from build123d import *

# Parameters (mm, degrees)
SKETCH1_W           = 38.1
SKETCH1_H           = 38.1
BOSS_EXTRUDE1_DEPTH = 7.62
SKETCH2_R           = 19.05
BOSS_EXTRUDE2_DEPTH = 25.4
SKETCH3_W           = 38.1
SKETCH3_H           = 38.1
BOSS_EXTRUDE3_DEPTH = 15.24
SKETCH4_R           = 6.296459426
BOSS_EXTRUDE4_DEPTH = 76.2
SKETCH5_W           = 3.175
SKETCH5_H           = 1.58699954
CUT_EXTRUDE1_DEPTH  = 73.66
SKETCH6_R           = 2.54
SKETCH6_R_2         = 2.5
CUT_EXTRUDE2_DEPTH  = 7.62
BOSS_EXTRUDE5_START = 71.374
SKETCH7_R           = 19.05
BOSS_EXTRUDE5_DEPTH = 71.374


with BuildPart() as part:
    # Sketch1 → Boss-Extrude1 (new body)
    with BuildSketch(Plane(origin=(0, 0, 0), x_dir=(1, 0, 0), z_dir=(0, 1, 0))):
        Rectangle(SKETCH1_W, SKETCH1_H)
    extrude(amount=BOSS_EXTRUDE1_DEPTH)

    # Sketch2 → Boss-Extrude2 (add)
    with BuildSketch(Plane(origin=(0, 7.62, 0), x_dir=(1, 0, 0), z_dir=(0, 1, 0))):
        with Locations(Location((0, 0, 0), (0, 0, 270))):
            Circle(SKETCH2_R)
    extrude(amount=BOSS_EXTRUDE2_DEPTH)

    # Sketch3 → Boss-Extrude3 (add)
    with BuildSketch(Plane(origin=(0, 33.02, 0), x_dir=(1, 0, 0), z_dir=(0, 1, 0))):
        Rectangle(SKETCH3_W, SKETCH3_H)
    extrude(amount=BOSS_EXTRUDE3_DEPTH)

    # Sketch4 → Boss-Extrude4 (add)
    with BuildSketch(Plane(origin=(0, 48.26, 0), x_dir=(1, 0, 0), z_dir=(0, 1, 0))):
        with Locations(Location((0, 0, 0), (0, 0, 90))):
            Circle(SKETCH4_R)
    extrude(amount=BOSS_EXTRUDE4_DEPTH)

    # Sketch5 → Cut-Extrude1 (cut)
    with BuildSketch(Plane(origin=(0, 124.46, 0), x_dir=(1, 0, 0), z_dir=(0, 1, 0))):
        with Locations((0, 6.38149977)):
            Rectangle(SKETCH5_W, SKETCH5_H)
    extrude(amount=-CUT_EXTRUDE1_DEPTH, mode=Mode.SUBTRACT)

    # Fillet1: read off the stored shape, not the designer's step
    # Fillet1 outline → Fillet1 (revolve, cut)
    with BuildSketch(Plane.XY):
        with BuildLine():
            ThreePointArc((5.026459426, 124.46), (5.924485038, 124.088025612), (6.296459426, 123.19))
            Line((6.296459426, 123.19), (6.296459426, 124.46))
            Line((6.296459426, 124.46), (5.026459426, 124.46))
        make_face()
    revolve(axis=Axis((0, 0, 0), (0, 1, 0)), mode=Mode.SUBTRACT)

    # Sketch6 → Cut-Extrude2 (cut)
    with BuildSketch(Plane(origin=(0, 0, -19.05), x_dir=(-1, 0, 0), z_dir=(0, 0, -1))):
        with Locations((-9.525, 3.81)):
            Circle(SKETCH6_R)
        with Locations((-9.525, 40.64)):
            Circle(SKETCH6_R)
        with Locations((9.525, 40.64)):
            Circle(SKETCH6_R)
        with Locations((9.525, 3.81)):
            Circle(SKETCH6_R_2)
    cut_extrude2 = extrude(amount=-CUT_EXTRUDE2_DEPTH, mode=Mode.SUBTRACT)

    # Mirror1: Cut-Extrude2 across plane
    add(cut_extrude2.mirror(Plane.XY), mode=Mode.SUBTRACT)

    # Sketch7 → Boss-Extrude5 (add)
    with BuildSketch(Plane.XZ.offset(BOSS_EXTRUDE5_START)):
        with Locations(Location((0, 0, 0), (0, 0, 270))):
            Circle(SKETCH7_R)
    extrude(amount=-BOSS_EXTRUDE5_DEPTH)


solid = part.part
The listing builds one solid part. Answer for the finished solid, in the listing's coordinates (mm). A direction names the side the tool comes from. Coordinates: 2 decimals unless noted, no trailing zeros. Write each loop counter-clockwise with the first axis right and the second up, starting at its lowest first coordinate (ties: lowest second). Pieces come first, ordered by that corner, then holes. Notation, with made-up numbers: M 81.5,28 L 99.5,28 A24 ccw 99.5,51 Z; hole C 48,83 d6. An arc over 180 degrees is marked long. Put each result on its own line as item: value. Start each with the question number.
1. A cutting plane is placed at C-C on y = 40.64. Write down the section's boundary in (x, z) (3 decimals), then the cut area to 3 significant figures.
2. Consider line 1 (Y direction, x = -9.5, z = -12.5); line 2 (X direction, y = 40, z = -13); line 3 (Y direction, x = -9, z = 5). Determine where each line is inside the solid, lowest interval first. Write a range as from..to.
3. Flat-ended cylindrical pins translate along their axes: P1, Ø4.5, axis at x = -9.525, y = 3.81, coming from the -Z side; P2, Ø1, axis at x = 8.5, z = -2, coming from the +Y side; P3, Ø12, axis at x = 5, y = 63, coming from the -Z side. Find the tip coordinate at first contact, or state that the pin passes through.
4. Which of the six approach directions +Z, -Z, +X, -X, +Y, -Y give full straight-line access (tool end or side, diameter ignored) to faces 1 (the cylindrical face through (-11.59, -36.19, 15.12)), 2 (the flat face through (-9, 41, 11.43)), 3 (the flat face through (14, 33.02, -15)), 4 (the cylindrical face through (8.16, 42.78, -15.29)), 5 (the flat face through (15, 33.02, 15))?
5. A cutting plane is placed at B-B on z = -15.5. Write down the section's boundary in (x, y) (3 decimals), then the cut area to 3 significant figures.
6. A cutting plane is placed at D-D on y = -53.5. Write down the section's boundary in (x, z).
7. For a pull along X with two mould halves and no side action, classify faces 6 (the flat face through (10, 41, -11.43)), 7 (the cylindrical face through (-11.59, 20.14, -15.12)), 8 (the flat face through (0, 124.46, 0)) as pulls with the +X half, pulls with the -X half, needs draft (parallel to the pull), parting line crosses it, or undercut.
8. A cutting plane is placed at A-A on y = 3.81. Write down the section's boundary in (x, z) (3 decimals).
Resolved:
1. outline: M -19.05,-19.05 L -12.065,-19.05 L -12.065,-11.43 L -6.985,-11.43 L -6.985,-19.05 L 6.985,-19.05 L 6.985,-11.43 L 12.065,-11.43 L 12.065,-19.05 L 19.05,-19.05 L 19.05,19.05 L 12.065,19.05 L 12.065,11.43 L 6.985,11.43 L 6.985,19.05 L -6.985,19.05 L -6.985,11.43 L -12.065,11.43 L -12.065,19.05 L -19.05,19.05 Z
1. area: 1,300 mm2
2. line 1: y = -71.37..1.31, 6.31..38.1, 43.18..48.26
2. line 2: x = -19.05..-11.98, -7.07..7.07, 11.98..19.05
2. line 3: y = -71.37..48.26
3. P1: stops at z = -11.43
3. P2: stops at y = 48.26
3. P3: stops at z = -6.09
4. face 1: -Y
4. face 2: +Z
4. face 3: -Z, +X
4. face 4: -Z
4. face 5: +Z, +X
5. outline: M -19.05,0 L -11.075,0 L -11.075,-71.374 L 11.075,-71.374 L 11.075,0 L 19.05,0 L 19.05,7.62 L 11.075,7.62 L 11.075,33.02 L 19.05,33.02 L 19.05,48.26 L -19.05,48.26 L -19.05,33.02 L -11.075,33.02 L -11.075,7.62 L -19.05,7.62 Z; hole C -9.525,40.64 d5.08; hole C -9.525,3.81 d5; hole C 9.525,3.81 d5.08; hole C 9.525,40.64 d5.08
5. area: 2,930 mm2
6. outline: C 0,0 d38.1
7. face 6: undercut
7. face 7: parting line crosses it
7. face 8: needs draft
8. outline: M -19.05,-19.05 L -12.025,-19.05 L -12.025,-11.43 L -7.025,-11.43 L -7.025,-19.05 L 6.985,-19.05 L 6.985,-11.43 L 12.065,-11.43 L 12.065,-19.05 L 19.05,-19.05 L 19.05,19.05 L 12.065,19.05 L 12.065,11.43 L 6.985,11.43 L 6.985,19.05 L -7.025,19.05 L -7.025,11.43 L -12.025,11.43 L -12.025,19.05 L -19.05,19.05 Z
